Could you check a few things on this model? Use its own coordinates, in mm. A direction names the side the tool comes from. Coordinates: 2 decimals unless noted, no trailing zeros. Loops run counter-clockwise (first coordinate to the right, second up) from the corner with the lowest first, then second, coordinate; pieces in that order, holes last. Notation, with made-up numbers: M 38.5,89.25 L 83.5,89.25 A11 cw 83.5,109.25 Z; hole C -35.75,18.5 d11. An arc over 180 degrees is marked long. Return JSON: item names as keys, results as strings. Group by question number.
from build123d import *

# Parameters (mm, degrees)
F0_R     = 9.525
F1_DEPTH = 12.7
F3_DEPTH = 47.498
F4_DEPTH = 31.75


# Not quite as in the source:
# - a feature names something its author has since deleted; it is built from what else it names


with BuildPart() as f1:
    # F0 (on Top) → F1 (new body)
    with BuildSketch(Plane.XY):
        Polygon((68.1566672574, 0), (-52.4933327426, 0), (-52.4933327426, -31.75), (-14.3933327426, -69.85), (30.0566672574, -69.85), (68.1566672574, -31.75), align=None)
        with Locations((-33.4641109884, -16.8546829373)):
            Circle(F0_R, mode=Mode.SUBTRACT)
        with Locations((49.0858890116, -16.5274422616)):
            Circle(F0_R, mode=Mode.SUBTRACT)
    extrude(amount=F1_DEPTH)

    # F2 (on Front) → F3 (join)
    with BuildSketch(Plane.XZ):
        Polygon((-14.398525469, 37.846), (-14.3439900845, 0), (30.1060099155, 0), (30.1060099155, 25.4), (0, 25.4), (0, 37.846), align=None)
    extrude(amount=F3_DEPTH)

    # F2 (on Front) → F4 (join)
    with BuildSketch(Plane.XZ):
        Polygon((-14.398525469, 56.896), (-14.398525469, 37.846), (0, 37.846), (0, 47.498), (30.051474531, 47.498), (30.051474531, 56.896), align=None)
    extrude(amount=F4_DEPTH)


solid = f1.part
(1) We'd pull the mould along Z, two halves only. Please class faces 6 (the face through (15, -23, 25.4)), 7 (the face through (3, -31.75, 50)), 8 (the face through (7, -34, 0)), 9 (the face through (0, -18, 36)): +Z half, -Z half, draft (parallel to the pull), parting line (faces both ways), or undercut.
(2) Imagine slicing it at D-D, the plane x = -9.5. Write out the boundary of the cut face in (y, z).
(3) Imagine slicing it at C-C, the plane z = 7. Write out the boundary of the cut face in (x, y) (3 decimals), then the cut area to 3 significant figures.
(4) If I drill on L1, parallel to Z at x = 22, y = -5.5; L2, parallel to X at y = -41.5, z = 18; L3, parallel to Z at x = 3, y = -34, over which ranges is the centre line in solid material (lowest first)? Write a range as [from, to].
(5) Will these pins go through, and if not, where does the flat tip stop? P1, Ø3, axis at y = -12.5, z = 51.5, coming from the +X side; P2, Ø8, axis at x = -17.5, z = 38, coming from the +Y side; P3, Ø10, axis at y = -61.5, z = 16, coming from the +X side; P4, Ø17, axis at x = -33.46, y = -16.85, coming from the +Z side.
(6) For faces 1 (the face through (-7, -40, 37.846)), 2 (the face through (-14.399, -16, 48)), 3 (the face through (15, -16, 47.498)), 4 (the face through (47.021, -25.826, 6.261)), 5 (the face through (30.051, -16, 52)), which set-ups out of +Z, -Z, +X, -X, +Y, -Y let a thin tool reach every point of the face, with its end or its side?
(7) Imagine slicing it at A-A, the plane x = 20. Write out the boundary of the cut face in (y, z).
(8) Imagine slicing it at B-B, the plane y = -12. Write out the boundary of the cut face in (x, z), then the cut area to 3 significant figures.
Checks:
{
 "1": {"face 6": "undercut", "face 7": "draft", "face 8": "-Z half", "face 9": "undercut"},
 "2": {"outline": "M -69.85,0 L 0,0 L 0,56.9 L -31.75,56.9 L -31.75,37.85 L -47.5,37.85 L -47.5,12.7 L -69.85,12.7 Z"},
 "3": {"outline": "M -52.493,-31.75 L -14.393,-69.85 L 30.057,-69.85 L 68.157,-31.75 L 68.157,0 L -52.493,0 Z; hole C -33.464,-16.855 d19.05; hole C 49.086,-16.527 d19.05", "area": "6,410 mm²"},
 "4": {"L1": "[0, 25.4], [47.5, 56.9]", "L2": "[-14.37, 30.11]", "L3": "[0, 25.4]"},
 "5": {"P1": "x = 30.05", "P2": "y = 0", "P3": "x = 42.16", "P4": "through"},
 "6": {"face 1": "+Z, +X, -X, -Y", "face 2": "+Z, -X, +Y, -Y", "face 3": "+X, +Y, -Y", "face 4": "+Z, -Z", "face 5": "+Z, +X, +Y, -Y"},
 "7": {"outline": "M -69.85,0 L 0,0 L 0,25.4 L -47.5,25.4 L -47.5,12.7 L -69.85,12.7 Z; M -31.75,47.5 L 0,47.5 L 0,56.9 L -31.75,56.9 Z"},
 "8": {"outline": "M -52.49,0 L -41.66,0 L -41.66,12.7 L -52.49,12.7 Z; M -25.27,0 L 40.71,0 L 40.71,12.7 L 30.11,12.7 L 30.11,25.4 L 0,25.4 L 0,47.5 L 30.05,47.5 L 30.05,56.9 L -14.4,56.9 L -14.4,37.85 L -14.36,12.7 L -25.27,12.7 Z; M 57.47,0 L 68.16,0 L 68.16,12.7 L 57.47,12.7 Z", "area": "2,410 mm²"}
}
